Geometry: see drawing. Coordinates: mm, zero at the bounding-box minimum. Coordinates: 2 decimals unless noted, no trailing zeros. Loops run counter-clockwise (first coordinate to the right, second up) from the corner with the lowest first, then second, coordinate; pieces in that order, holes last. Notation, with made-up numbers: (85.5, -5.75) -> (126.5, -5.75) arc R18 ccw to (126.5, 2.25) -> close; hole circle Ø3 at (77.5, -0.5). An arc over 180 degrees is marked (long way). One line per question, with ' | ' between items. Start each with the question number.
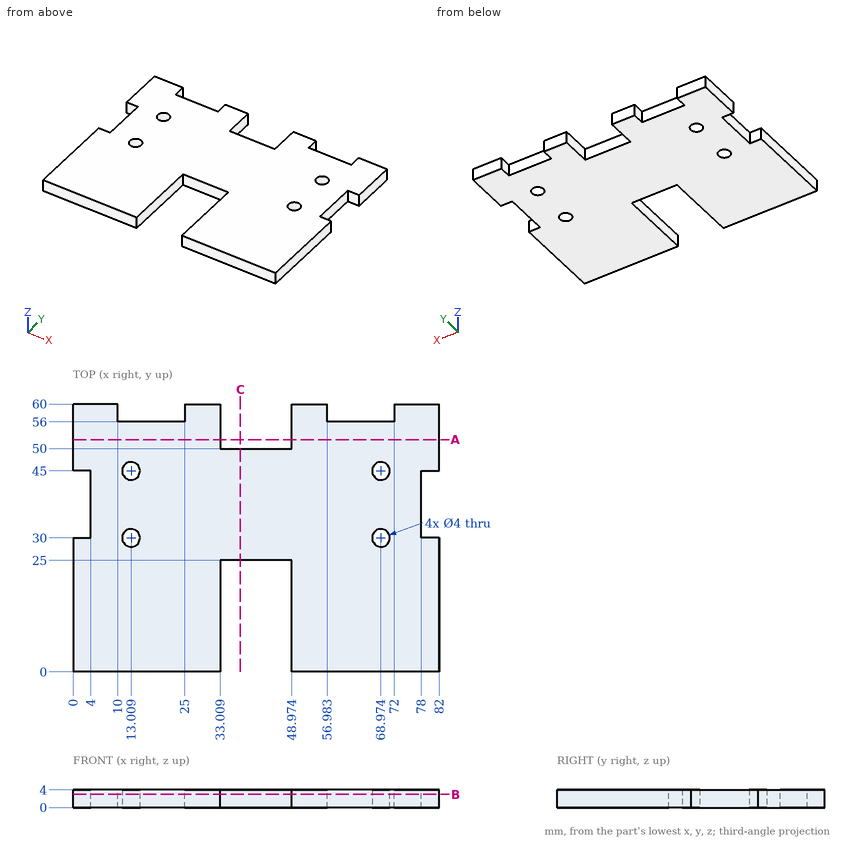
(1) Ray query, L1, parallel to X at y = 5.5, z = 1.5; L2, parallel to Y at x = 14, z = 1; L3, parallel to Y at x = 22, z = 3.5. Return the intervals inside material, ascending.
(2) Cut plane A-A, the plane y = 52. Return the cut outline in (x, z).
(3) Cut plane B-B, the plane z = 3. State how many separate pieces and enclosed holes the cut face has, and give its area (3 significant figures).
(4) Contact query for flat-ended pins moving along their axis: pin 1 Ø2.5 at (x, y) = (68.97, 30) entering from +Z; pin 2 Ø5 at (x, y) = (18.5, 24) entering from -Z; pin 3 Ø2 at (x, z) = (62, 1.5) entering from +Y; pin 4 Ø1 at (y, z) = (38.5, 3.5) entering from -X. Output: stop coordinate, or through.
(5) Cut plane C-C, the plane x = 37.5. Return the cut outline in (y, z).
Here are the results:
1) L1: x = 0 to 33.01, 48.97 to 82 | L2: y = 0 to 28.26, 31.74 to 43.26, 46.74 to 56 | L3: y = 0 to 56
2) outline: (0, 0) -> (33.01, 0) -> (33.01, 4) -> (0, 4) -> close; (48.97, 0) -> (82, 0) -> (82, 4) -> (48.97, 4) -> close
3) separate pieces: 1 | enclosed holes: 4 | area: 4,070 mm2
4) pin 1: passes through | pin 2: stops at z = 0 | pin 3: stops at y = 56 | pin 4: stops at x = 4
5) outline: (25, 0) -> (50, 0) -> (50, 4) -> (25, 4) -> close
